CAD build for the part. Positions are in the model's coordinates, mm. A direction names the side the tool comes from. Give positions to 0.01 mm unless a question says otherwise; leave off trailing zeros. Order: outer loops, then holes, each group sorted by start corner. A loop starts at its lowest first (then second) coordinate and runs counter-clockwise, first axis right, second up. Notation, with made-up numbers: M 62.25,68.25 L 89.25,68.25 A24 ccw 89.25,89.25 Z; hole C 67,62.5 d9. An arc over 180 degrees is marked long. Put each result on its own line as item: value. Start each with the question number.
1) Cut at A-A (y = 8.75). Write the cut outline in (x, z), and give its area (3 significant figures).
2) Two-plate mould, pull along X, no slides. Class faces 4 (the face through (3.412, 6.153, -4.287)), 5 (the face through (1.802, 5.346, 5.723)), 6 (the face through (-0.098, 11.594, -4.891)), 7 (the face through (0, 5.5, 0)): released by +X, released by -X, zero draft, split by the parting line, or undercut.
3) Cut at B-B (x = 0.5). Write the cut outline in (y, z), and give its area (3 significant figures).
4) Cut at C-C (z = 4.5). Write the cut outline in (x, y), and give its area (3 significant figures).
5) Drill centre lines: line 1 (Y direction, x = 0, z = 4.75); line 2 (Y direction, x = 3.5, z = -2); line 3 (X direction, y = 10.85, z = -4.5). Where is each one in solid material? Low to high. Write a range as [from, to].
6) Tool access for faces 1 (the face through (-3.15, 9, 4)), 2 (the face through (3.15, 9, 4)), 3 (the face through (-0.1, 9.7, 3.75)): list every direction of +Z, -Z, +X, -X, +Y, -Y with a clear straight run to the whole face (end or side of a thin tool).
7) Cut at D-D (z = 0). Write the cut outline in (x, y), and give its area (3 significant figures).
8) Pin check, flat tips, straight feed: pin 1 (3 mm diameter, centred on x = -4, z = -1.5, fed in from -Y); pin 2 (1 mm diameter, centred on x = -3, z = -4.5, fed in from +Y); pin 3 (4 mm diameter, centred on x = -0.5, z = 0, fed in from +Y); pin 4 (1.5 mm diameter, centred on y = 8.5, z = 4.5, fed in from +X). Stop position of each tip, or through.
```python
from build123d import *

# Parameters (mm, degrees)
SKETCH1_R               = 6
BOSS_EXTRUDE1_DEPTH     = 14
CUT_EXTRUDE1_DEPTH      = 17.370705544
CUT_EXTRUDE1_DEPTH_BACK = 17.370705544
SKETCH2_W               = 7.5
SKETCH2_H               = 8.5
CUT_EXTRUDE2_DEPTH      = 17.370705544
CUT_EXTRUDE2_DEPTH_BACK = 17.370705544
SKETCH3_R               = 0.75


with BuildPart() as part:
    # Sketch1 → Boss-Extrude1 (new body)
    with BuildSketch(Plane(origin=(0, 0, 0), x_dir=(1, 0, 0), z_dir=(0, 1, 0))):
        with Locations(Location((0, 0, 0), (0, 0, 270))):
            Circle(SKETCH1_R)
    extrude(amount=BOSS_EXTRUDE1_DEPTH)

    # Sketch2 → Cut-Extrude1 (cut, two sides: drawn at the far end of the back side and taken through both)
    with BuildSketch(Plane(origin=(0, 0, 0), x_dir=(0, 0, -1), z_dir=(1, 0, 0)).offset(-CUT_EXTRUDE1_DEPTH_BACK)):
        with Locations((0, 9.75)):
            Rectangle(SKETCH2_W, SKETCH2_H)
    extrude(amount=CUT_EXTRUDE1_DEPTH + CUT_EXTRUDE1_DEPTH_BACK, mode=Mode.SUBTRACT)

    # Sketch3 → Cut-Extrude2 (cut, two sides: drawn at the far end of the back side and taken through both)
    with BuildSketch(Plane.XY.offset(-CUT_EXTRUDE2_DEPTH_BACK)):
        with BuildLine():
            Line((-3.15, 7), (-3.15, 10.85))
            ThreePointArc((-3.15, 10.85), (-2.227386361, 13.077386361), (0, 14))
            Line((0, 14), (-4.683748499, 14))
            Line((-4.683748499, 14), (-4.683748499, 5.5))
            Line((-4.683748499, 5.5), (-4.65, 5.5))
            ThreePointArc((-4.65, 5.5), (-3.589339828, 5.939339828), (-3.15, 7))
        make_face()
        with BuildLine():
            Line((4.683748499, 14), (0, 14))
            ThreePointArc((0, 14), (2.227386361, 13.077386361), (3.15, 10.85))
            Line((3.15, 10.85), (3.15, 7))
            ThreePointArc((3.15, 7), (3.589339828, 5.939339828), (4.65, 5.5))
            Line((4.65, 5.5), (4.683748499, 5.5))
            Line((4.683748499, 5.5), (4.683748499, 14))
        make_face()
        with Locations((0, 10.85)):
            Circle(SKETCH3_R)
    extrude(amount=CUT_EXTRUDE2_DEPTH + CUT_EXTRUDE2_DEPTH_BACK, mode=Mode.SUBTRACT)


solid = part.part
```
Solution:
1. outline: M -3.15,-5.11 A6 ccw 3.15,-5.11 L 3.15,-3.75 L -3.15,-3.75 Z; M -3.15,3.75 L 3.15,3.75 L 3.15,5.11 A6 ccw -3.15,5.11 Z
1. area: 24.7 mm²
2. face 4: released by +X
2. face 5: split by the parting line
2. face 6: undercut
2. face 7: zero draft
3. outline: M 0,-5.98 L 10.29,-5.98 L 10.29,-3.75 L 5.5,-3.75 L 5.5,3.75 L 10.29,3.75 L 10.29,5.98 L 0,5.98 Z; M 11.41,-5.98 L 13.96,-5.98 L 13.96,-3.75 L 11.41,-3.75 Z; M 11.41,3.75 L 13.96,3.75 L 13.96,5.98 L 11.41,5.98 Z
3. area: 98.5 mm²
4. outline: M -3.97,0 L 3.97,0 L 3.97,5.66 A1.5 cw 3.15,7 L 3.15,10.85 A3.15 ccw -3.15,10.85 L -3.15,7 A1.5 cw -3.97,5.66 Z; hole C 0,10.85 d1.5
4. area: 92.1 mm²
5. line 1: [0, 10.1], [11.6, 14]
5. line 2: [0, 5.5]
5. line 3: [-3.15, -0.75], [0.75, 3.15]
6. face 1: +Z, -Z, -X, +Y
6. face 2: +Z, -Z, +X, +Y
6. face 3: +X, -X, +Y
7. outline: M -6,0 L 6,0 L 6,5.5 L -6,5.5 Z
7. area: 66.0 mm²
8. pin 1: y = 0
8. pin 2: y = 12.77
8. pin 3: y = 5.5
8. pin 4: x = 3.15
